Can you work these out from the model? Positions are in its coordinate system, mm. Give positions to 0.01 mm unless a question says otherwise; leave off trailing zeros. Write each loop counter-clockwise with the first axis right and the second up, starting at its lowest first coordinate (ties: lowest second). Pieces come first, ordered by that corner, then holes. Notation, with made-up numbers: M -23,39.25 L 8,39.25 A19 cw 8,46.25 Z; hole C 85.5,-7.75 d11. An arc over 180 degrees is marked long. Write each question's results on one line, items separated by ' | '.
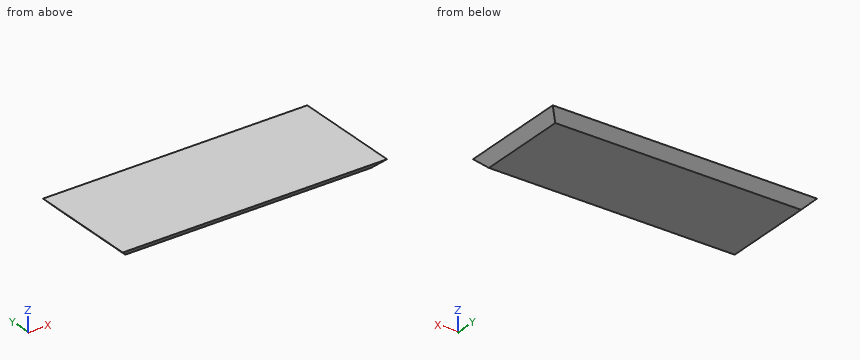
from build123d import *

# Parameters (mm, degrees)
F0_W     = 630
F0_H     = 263
F1_DEPTH = 22
F2_SIZE  = 21.99999


# Not quite as in the source:
# - a fillet or chamfer is up to 0.001 mm smaller than in the source, because OpenCascade refuses the exact size


with BuildPart() as f1:
    # F0 (on Top) → F1 (new body)
    with BuildSketch(Plane.XY):
        Rectangle(F0_W, F0_H)
    extrude(amount=F1_DEPTH)

    # F2 (size 22 in the source; OpenCascade refuses exactly that, so slightly less here)
    f2_edges = [f1.edges().sort_by_distance(p)[0] for p in [
        (0, 131.5, 0),
        (315, 0, 0),
        (0, -131.5, 0),
        (-315, 0, 0),
    ]]
    chamfer(f2_edges, length=F2_SIZE)


solid = f1.part
Item 1: If I drill on line 1 (X direction, y = 54, z = 19.5); line 2 (X direction, y = -61.5, z = 9.25); line 3 (Y direction, x = 120, z = 11.75), over which ranges is the centre line in solid material (lowest first)? Write a range as from..to.
Geometry says:
line 1: x = -312.5..312.5 | line 2: x = -302.25..302.25 | line 3: y = -121.25..121.25
Item 2: I want a section at C-C, the plane z = 5. Please give me the cut outline in (x, y).
Geometry says:
outline: M -298,-114.5 L 298,-114.5 L 298,114.5 L -298,114.5 Z
Item 3: I'm going to push flat-ended pins straight in: pin 1 (2 mm diameter, centred on x = -227, z = 17.5, fed in from -Y); pin 2 (8 mm diameter, centred on y = -64, z = 3.5, fed in from -X); pin 3 (1.5 mm diameter, centred on y = -47.5, z = 8, fed in from +X). Where does each tip first touch, or does it pass through?
Geometry says:
pin 1: stops at y = -128 | pin 2: stops at x = -300.5 | pin 3: stops at x = 301.75
